Check sheet for the drawn part. Datum: minimum x, y, z corner. Units: mm. A direction names the side the tool comes from. Give positions to 0.01 mm unless a question says otherwise; leave off trailing zeros. Order: outer loops, then holes, each group sorted by start corner. A loop starts at its lowest first (then second) coordinate and runs counter-clockwise, first axis right, second up. Notation, with made-up numbers: (8.25, 10.5) -> (58.25, 10.5) arc R5 ccw to (58.25, 17.5) -> close; hole circle Ø3 at (-10.5, 43.5). An arc over 180 degrees is marked (long way). Return JSON: item names as keys, results as strings. Group by question number.
(1) Cross-section at B-B on z = 10.5. Enter the section's corners in (x, y), then the cut area to 3 significant figures.
(2) Cross-section at A-A on x = 4. State how many separate pieces and enclosed holes the cut face has, then the cut area to 3 significant figures.
(3) Thickness scan on line 1 along Y through (x, z) = (18.45, 4); line 2 along Y through (x, z) = (4, 12); line 3 along Y through (x, z) = (1.55, 12). Record the ranges inside material, lowest first.
(4) Cross-section at C-C on y = 14. Enter the section's corners in (x, z), then the cut area to 3 significant figures.
(5) Depth check by flat-ended pin: pin 1 Ø2.5 at (y, z) = (36, 4) entering from -X; pin 2 Ø5 at (x, y) = (24, 14) entering from -Z; pin 3 Ø12 at (x, y) = (14, 5.5) entering from +Z; pin 4 Ø6 at (x, z) = (20.5, 2) entering from -Y. Enter the tip coordinate at first touch or a pass-through.
(6) Tool access check on the marked faces 4 and 5. Record the directions out of +Z, -Z, +X, -X, +Y, -Y that give a thin tool (end or side, any length) a straight path to the whole face; none if there is none.
(7) Cross-section at D-D on z = 7. Enter the section's corners in (x, y).
(8) Release check for a two-part mould opening along Z. For the marked faces 1, 2 and 3 record: pulls with the +Z half, pulls with the -Z half, needs draft (parallel to the pull), parting line crosses it, or undercut.
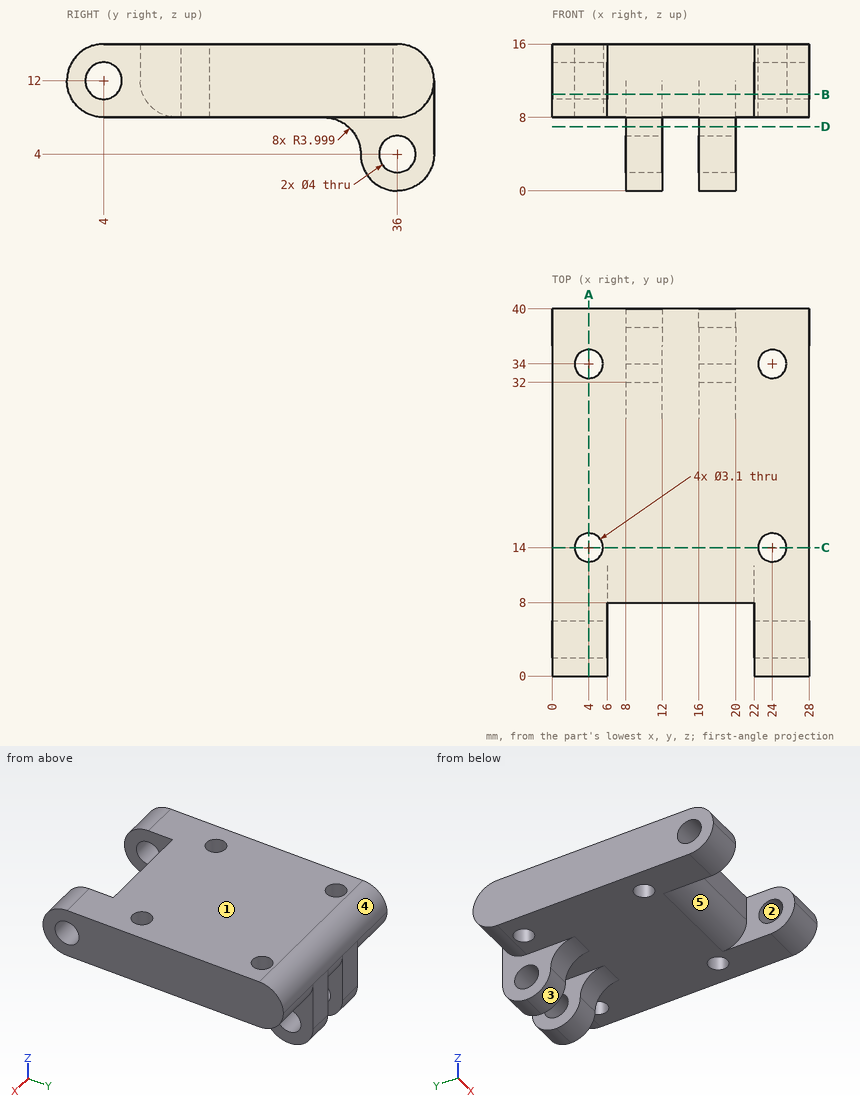
Verdict:
{
 "1": {"outline": "(0, 0.29) -> (6, 0.29) -> (6, 2.68) -> (0, 2.68) -> close; (0, 5.32) -> (6, 5.32) -> (6, 8.29) -> (22, 8.29) -> (22, 5.32) -> (28, 5.32) -> (28, 39.71) -> (20, 39.71) -> (20, 40) -> (16, 40) -> (16, 39.71) -> (12, 39.71) -> (12, 40) -> (8, 40) -> (8, 39.71) -> (0, 39.71) -> close; (22, 0.29) -> (28, 0.29) -> (28, 2.68) -> (22, 2.68) -> close; hole circle Ø3.1 at (4, 14); hole circle Ø3.1 at (4, 34); hole circle Ø3.1 at (24, 14); hole circle Ø3.1 at (24, 34)", "area": "916 mm²"},
 "2": {"separate pieces": "3", "enclosed holes": "1", "area": "244 mm²"},
 "3": {"line 1": "32 to 34, 38 to 40", "line 2": "0 to 2, 6 to 12.45, 15.55 to 32.45, 35.55 to 40", "line 3": "0 to 2, 6 to 40"},
 "4": {"outline": "(0, 8) -> (2.45, 8) -> (2.45, 16) -> (0, 16) -> close; (5.55, 8) -> (22.45, 8) -> (22.45, 16) -> (5.55, 16) -> close; (25.55, 8) -> (28, 8) -> (28, 16) -> (25.55, 16) -> close", "area": "174 mm²"},
 "5": {"pin 1": "through", "pin 2": "z = 8", "pin 3": "z = 16", "pin 4": "y = 31.88"},
 "6": {"face 4": "+Z, +X, -X, +Y", "face 5": "-Z, -Y"},
 "7": {"outline": "(8, 30.65) -> (12, 30.65) -> (12, 40) -> (8, 40) -> close; (16, 30.65) -> (20, 30.65) -> (20, 40) -> (16, 40) -> close"},
 "8": {"face 1": "pulls with the +Z half", "face 2": "undercut", "face 3": "pulls with the -Z half"}
}
